Read the model definition and answer for the solid it produces. Units are mm, in the model's axes. Coordinates: 2 decimals unless noted, no trailing zeros. Loops run counter-clockwise (first coordinate to the right, second up) from the corner with the lowest first, then second, coordinate; pieces in that order, holes last.
Autodesk Fusion 360 part; units mm, degrees
sketch "Sketch1" plane through (0, 0, 0) normal (0, 1, 0) x (1, 0, 0)
  line L0 (0, 0) -> (38.5, 0)
  line L1 (38.5, 0) -> (38.5, -38.5)
  line L2 (38.5, -38.5) -> (0, -38.5)
  line L3 (0, -38.5) -> (0, 0)
  circle A0 centre (20, -20) radius 13
  dimension "d1" = 38.5
  dimension "d2" = 38.5
  dimension "d3" = 26
extrude "Extrude1" add sketch "Sketch1" along normal blind 1.5
Item 1: Find the intervals of material crossed by line 1 along Z through (x, y) = (20, 0.6); line 2 along Z through (x, y) = (14, 1.4), in increasing order.
Numbers:
line 1: z = 0 to 7, 33 to 38.5
line 2: z = 0 to 8.47, 31.53 to 38.5
Item 2: Determine the mould class of faces 1 (the face through (32.4, 0.7, 23.9)), 2 (the face through (19, 1, 0)), 3 (the face through (38.5, 1, 19)) for opening direction X: released by +X, released by -X, zero draft, split by the parting line, or undercut.
Numbers:
face 1: undercut
face 2: zero draft
face 3: released by +X
Item 3: A cutting plane is placed at A-A on x = 20. Determine the outline of the cut face in (y, z).
Numbers:
outline: (0, 0) - (1.5, 0) - (1.5, 7) - (0, 7) - close; (0, 33) - (1.5, 33) - (1.5, 38.5) - (0, 38.5) - close
Item 4: A cutting plane is placed at B-B on z = 20. Determine the outline of the cut face in (x, y).
Numbers:
outline: (0, 0) - (7, 0) - (7, 1.5) - (0, 1.5) - close; (33, 0) - (38.5, 0) - (38.5, 1.5) - (33, 1.5) - close
Item 5: A cutting plane is placed at C-C on y = 1.05. Determine the outline of the cut face in (x, z).
Numbers:
outline: (0, 0) - (38.5, 0) - (38.5, 38.5) - (0, 38.5) - close; hole circle Ø26 at (20, 20)
